Autodesk Inventor part; units mm, degrees
ref_plane "WorkPlane1" through (0, 0, 0) normal (0, 0, 1) x (1, 0, 0)
ref_plane "Work Plane2" through (0, 0, -1) normal (0, 0, 1) x (1, 0, 0)
ref_plane "WorkPlane2" through (0, 0, 1.5) normal (0, 0, 1) x (1, 0, 0)
ref_plane "WorkPlane1" through (0, 0, 0) normal (0, 0, 1) x (1, 0, 0)
ref_plane "Work Plane2" through (0, 0, -1) normal (0, 0, 1) x (1, 0, 0)
ref_plane "WorkPlane2" through (0, 0, 1.5) normal (0, 0, 1) x (1, 0, 0)
sketch "Sketch1" plane through (0, 0, 0) normal (0, 0, 1) x (1, 0, 0)
  point P0 (0, 0)
sketch "Sketch2" plane through (0, 0, 0) normal (0, 0, 1) x (1, 0, 0)
  line L0 (3.75, -7.5121) -> (3.75, -4.65)
  line L1 (0.75, -8.041) -> (3.75, -7.5121)
  line L2 (0.75, -4.741) -> (0.75, -8.041)
  arc A0 (0.75, -4.741) -> (-0.75, -4.741) centre (0, 0) ccw
  line L3 (-0.75, -4.741) -> (-0.75, -8.041)
  line L4 (-0.75, -8.041) -> (-3.75, -7.5121)
  line L5 (-3.75, -7.5121) -> (-3.75, -4.65)
  arc A1 (3.75, -4.65) -> (-3.75, -4.65) centre (0, 0.35) ccw
  dimension "d2" = 4.8
  dimension "d4" = 6.25
  dimension "d6" = 0
  dimension "d8" = 0.75
  dimension "d10" = 0.75
  dimension "d12" = 3.3
  dimension "d14" = 3.3
  dimension "d16" = 80
  dimension "d18" = 80
  dimension "d20" = 3
  dimension "d22" = 3
  dimension "d24" = 0.35
  dimension "d52" = 0
  dimension "d53" = 0
extrude "Extrusion1" add sketch "Sketch2" along normal blind 1
sketch "Sketch3" plane through (0, 0, 1) normal (0, 0, 1) x (1, 0, 0)
  line L0 (-0.75, -4.741) -> (-0.75, -8.041)
  line L1 (-0.75, -8.041) -> (-3.75, -7.5121)
  point P0 (-1.95, -6.3215)
  dimension "d30" = 1.2
  dimension "d32" = 1.485
hole "Hole1" at (-1.95, -6.3215, 1) direction (0, 0, -1) diameter 1.5 end through all
sketch "Sketch4" plane through (0, 0, 1) normal (0, 0, 1) x (1, 0, 0)
  line L0 (0.75, -8.041) -> (0.75, -4.741)
  line L1 (3.75, -7.5121) -> (0.75, -8.041)
  point P0 (1.95, -6.3215)
  dimension "d41" = 1.2
  dimension "d43" = 1.485
hole "Hole2" at (1.95, -6.3215, 1) direction (0, 0, -1) diameter 1.5 end through all
fillet "Fillet1" radius 2.25 2 edges at (-3.75, -7.5121, 0.5) (3.75, -7.5121, 0.5)
equation "\"d33\" = Diam5"
equation "\"d44\" = Diam5"
equation "\"d51\" = 1.5 * Diam5"
equation "\"d2\" = 0.5 * Diam2"
equation "\"d4\" = 0.166667 * ParA + 0.5 * Diam2 + 0.5 * b"
equation "\"d8\" = 0.5 * Diam5"
equation "\"d10\" = 0.5 * Diam5"
equation "\"d12\" = ParA"
equation "\"d14\" = ParA"
equation "\"d20\" = 2 * Diam5"
equation "\"d22\" = 2 * Diam5"
equation "\"d24\" = -msp_r2 + 0.5 * Diam2 + b"
equation "\"d25\" = ParS"
equation "\"Diam5\" = 1.5"
equation "\"ParA\" = 3.3"
equation "\"ParS\" = 1"
equation "\"Diam2\" = 9.6"
equation "\"msp_r2\" = 0.166667 * ParA + 0.5 * Diam2 + 0.5 * b"
equation "\"TEMPLATE\" = 1.2345"
properties part number "DIN 471 - 10x1" material "Steel, Mild"
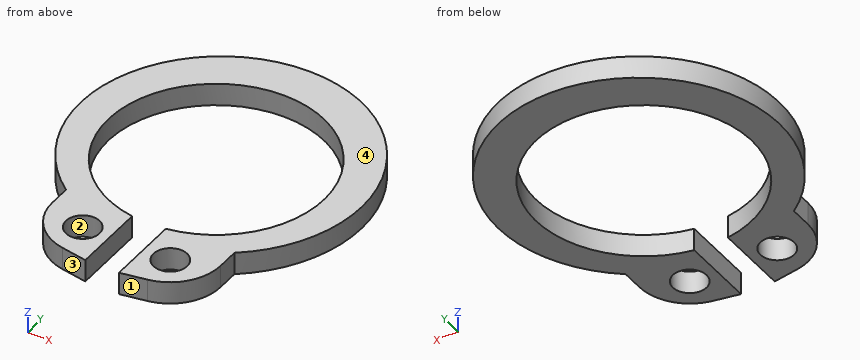
Work out the finished part from the listing and answer in its coordinate system (mm). Face numbers are marked on the shaded views. Round coordinates to 2 decimals unless told otherwise and drop trailing zeros. Write each loop counter-clockwise with the first axis right and the second up, starting at its lowest first coordinate (ties: lowest second). Pieces come first, ordered by that corner, then holes. Notation, with made-up numbers: (48, -31.75) - (96, -31.75) arc R32 ccw to (96, 3.25) - close; hole circle Ø1 at (73, 14.5). An arc over 180 degrees is marked (long way). Return JSON: item names as keys, results as strings. Group by question number.
Q1. The part is cut by section A-A on z = 0.85. Write down the section's boundary in (x, y).
Q2. The part is cut by section D-D on y = -6.5. Write down the section's boundary in (x, z).
Q3. The part is cut by section C-C on y = -2.5. Write down the section's boundary in (x, z), then the cut area to 3 significant figures.
Q4. The part is cut by section B-B on x = 1.5. Write down the section's boundary in (y, z).
Q5. Find the intervals of material crossed by L1, parallel to Y at x = 1.95, z = 0.65; L2, parallel to Y at x = 0, z = 0.85; L3, parallel to X at y = -2.75, z = 0.65, in increasing order.
Q6. The mould has two halves that part along X. Classify the marked faces 1, 2, 3 and 4: released by +X, released by -X, zero draft, split by the parting line, or undercut.
Q7. This flat-tipped pin is pushed along its axis until it touches: pin 1 Ø1.4 at (x, y) = (-1.95, -6.32) entering from -Z. Where does it stop, or does it pass through?
Solved:
{
 "1": {"outline": "(-3.75, -5.62) arc R2.25 ccw to (-1.89, -7.84) - (-0.75, -8.04) - (-0.75, -4.74) arc R4.8 cw (long way) to (0.75, -4.74) - (0.75, -8.04) - (1.89, -7.84) arc R2.25 ccw to (3.75, -5.62) - (3.75, -4.65) arc R6.25 ccw (long way) to (-3.75, -4.65) - close; hole circle Ø1.5 at (-1.95, -6.32); hole circle Ø1.5 at (1.95, -6.32)"},
 "2": {"outline": "(-3.57, 0) - (-2.68, 0) - (-2.68, 1) - (-3.57, 1) - close; (-1.22, 0) - (-0.75, 0) - (-0.75, 1) - (-1.22, 1) - close; (0.75, 0) - (1.22, 0) - (1.22, 1) - (0.75, 1) - close; (2.68, 0) - (3.57, 0) - (3.57, 1) - (2.68, 1) - close"},
 "3": {"outline": "(-5.56, 0) - (-4.1, 0) - (-4.1, 1) - (-5.56, 1) - close; (4.1, 0) - (5.56, 0) - (5.56, 1) - (4.1, 1) - close", "area": "2.93 mm²"},
 "4": {"outline": "(-7.91, 0) - (-6.92, 0) - (-6.92, 1) - (-7.91, 1) - close; (-5.72, 0) - (-4.56, 0) - (-4.56, 1) - (-5.72, 1) - close; (4.56, 0) - (6.42, 0) - (6.42, 1) - (4.56, 1) - close"},
 "5": {"L1": "-7.83 to -7.07, -5.57 to -4.39, 4.39 to 6.29", "L2": "4.8 to 6.6", "L3": "-5.43 to -3.93, 3.93 to 5.43"},
 "6": {"face 1": "released by +X", "face 2": "undercut", "face 3": "released by -X", "face 4": "zero draft"},
 "7": {"pin 1": "through"}
}
